Can you work these out from the model? Positions are in its coordinate system, mm. A direction names the side the tool comes from. Coordinates: 2 decimals unless noted, no trailing zeros. Loops run counter-clockwise (first coordinate to the right, second up) from the corner with the lowest first, then second, coordinate; pieces in that order, holes last. Notation, with made-up numbers: (64.5, 81.5) -> (86.5, 81.5) arc R16 cw to (86.5, 108.5) -> close; hole circle Ø3 at (31, -21.75). An arc over 180 degrees is marked (long way). Put each result on its own line as item: value. Start each with the question number.
Item 1: For faces 1 (the flat face through (39.57, 69, 3)), 2 (the flat face through (50, 69, 2)), which set-ups out of +Z, -Z, +X, -X, +Y, -Y let a thin tool reach every point of the face, with its end or its side?
Item 2: If we section it at A-A on y = 66.5: Please give me the cut outline in (x, z), plus the area to 3 significant figures.
Item 3: We'd pull the mould along Y, two halves only. Please class faces 3 (the cylindrical face through (17.26, 80.04, 2.47)), 4 (the cylindrical face through (47.15, 3.01, 2.54)), 5 (the flat face through (1, 71, 0)), 6 (the flat face through (1, 140, 2)): pulls with the +Y half, pulls with the -Y half, needs draft (parallel to the pull), parting line crosses it, or undercut.
Item 4: Will this pin go through, and if not, where does the flat tip stop? P1, Ø4, axis at x = -19.57, y = 57, coming from the +Z side (1 decimal).
Item 5: Please list where these lines run through material, in increasing order: L1, parallel to X at y = 71, z = 1.75; L2, parallel to X at y = 81.5, z = 2.95; L3, parallel to Y at x = 37, z = 1.65. Write a range as from..to.
Item 6: If we section it at C-C on y = 81: Please give me the cut outline in (x, z), plus the area to 3 significant figures.
Item 7: If we section it at B-B on z = 3.9: Please give me the cut outline in (x, y).
```python
from build123d import *

# Parameters (mm, degrees)
F0_W     = 50
F0_H     = 140
F1_DEPTH = 5
F4_DEPTH = 62.609963119
F6_D     = 5
F8_R     = 10
F9_R     = 10
F10_R    = 10
F11_R    = 10


with BuildPart() as f1:
    # F0 (on Top) → F1 (new body)
    with BuildSketch(Plane.XY):
        with Locations((25, 70)):
            Rectangle(F0_W, F0_H)
    extrude(amount=F1_DEPTH)

    # F3 (on face) → F4 (cut)
    with BuildSketch(Plane.XY.offset(5)):
        with BuildLine():
            ThreePointArc((34.5700508356, 45), (37.0700508356, 42.5), (39.5700508356, 45))
            Line((39.5700508356, 45), (39.5700508356, 93))
            ThreePointArc((39.5700508356, 93), (37.0700508356, 95.5), (34.5700508356, 93))
            Line((34.5700508356, 93), (34.5700508356, 45))
        make_face()
    extrude(amount=-F4_DEPTH, mode=Mode.SUBTRACT)

    # F6 (through all)
    with Locations(Plane.XY.offset(5)):
        with Locations((19.5700508356, 57), (19.5700508356, 81)):
            Hole(F6_D / 2)

    # F7: F1 across plane


with BuildPart() as f1_1:
    add(f1.part)
    add(f1.part.mirror(Plane.YZ))

    # F8
    f8_edges = [f1_1.edges().sort_by_distance(p)[0] for p in [
        (50, 140, 2.5),
    ]]
    fillet(f8_edges, radius=F8_R)

    # F9
    f9_edges = [f1_1.edges().sort_by_distance(p)[0] for p in [
        (50, 0, 2.5),
    ]]
    fillet(f9_edges, radius=F9_R)

    # F10
    f10_edges = [f1_1.edges().sort_by_distance(p)[0] for p in [
        (-50, 0, 2.5),
    ]]
    fillet(f10_edges, radius=F10_R)

    # F11
    f11_edges = [f1_1.edges().sort_by_distance(p)[0] for p in [
        (-50, 140, 2.5),
    ]]
    fillet(f11_edges, radius=F11_R)


solid = f1_1.part
```
Solutions:
1. face 1: +Z, -Z
1. face 2: +Z, -Z, +X, +Y, -Y
2. outline: (-50, 0) -> (-39.57, 0) -> (-39.57, 5) -> (-50, 5) -> close; (-34.57, 0) -> (34.57, 0) -> (34.57, 5) -> (-34.57, 5) -> close; (39.57, 0) -> (50, 0) -> (50, 5) -> (39.57, 5) -> close
2. area: 450 mm^2
3. face 3: undercut
3. face 4: pulls with the -Y half
3. face 5: needs draft
3. face 6: pulls with the +Y half
4. P1: through
5. L1: -50..-39.57, -34.57..34.57, 39.57..50
5. L2: -50..-39.57, -34.57..-22.02, -17.12..17.12, 22.02..34.57, 39.57..50
5. L3: 0..42.5, 95.5..140
6. outline: (-50, 0) -> (-39.57, 0) -> (-39.57, 5) -> (-50, 5) -> close; (-34.57, 0) -> (-22.07, 0) -> (-22.07, 5) -> (-34.57, 5) -> close; (-17.07, 0) -> (17.07, 0) -> (17.07, 5) -> (-17.07, 5) -> close; (22.07, 0) -> (34.57, 0) -> (34.57, 5) -> (22.07, 5) -> close; (39.57, 0) -> (50, 0) -> (50, 5) -> (39.57, 5) -> close
6. area: 400 mm^2
7. outline: (-50, 10) arc R10 ccw to (-40, 0) -> (40, 0) arc R10 ccw to (50, 10) -> (50, 130) arc R10 ccw to (40, 140) -> (-40, 140) arc R10 ccw to (-50, 130) -> close; hole (-39.57, 45) arc R2.5 ccw to (-34.57, 45) -> (-34.57, 93) arc R2.5 ccw to (-39.57, 93) -> close; hole circle Ø5 at (-19.57, 57); hole circle Ø5 at (-19.57, 81); hole circle Ø5 at (19.57, 57); hole circle Ø5 at (19.57, 81); hole (34.57, 45) arc R2.5 ccw to (39.57, 45) -> (39.57, 93) arc R2.5 ccw to (34.57, 93) -> close
